The model under review builds one solid part; all positions refer to its coordinate system, in mm. A direction names the side the tool comes from. Coordinates: 2 decimals unless noted, no trailing zeros. Order: outer loops, then holes, each group sorted by start corner. A loop starts at its lowest first (then second) coordinate and runs counter-clockwise, first axis right, second up. Notation, with made-up numbers: M 4.5,89.5 L 13.5,89.5 A27 ccw 13.5,120.5 Z; hole C 82.5,44 d9. An arc over 180 degrees is marked long. Answer in a Markdown table with one row per item.
Autodesk Inventor part; units mm, degrees
ref_plane "YZ Plane" through (0, 0, 0) normal (1, 0, 0) x (0, 1, 0)
ref_plane "XZ Plane" through (0, 0, 0) normal (0, 1, 0) x (-1, 0, 0)
ref_plane "XY Plane" through (0, 0, 0) normal (0, 0, 1) x (1, 0, 0)
sketch "Sketch1" plane through (0, 0, 0) normal (0, 1, 0) x (-1, 0, 0)
  circle A0 centre (0, 0) radius 18.4566
  circle A1 centre (10, 10) radius 2
  circle A2 centre (10, -10) radius 2
  circle A3 centre (-10, -10) radius 2
  circle A4 centre (-10, 10) radius 2
  point P0 (8.8496, 0)
extrude "Extrusion1" add sketch "Sketch1" along normal blind 10
sketch "Sketch2" plane through (0, 10, 0) normal (0, 1, 0) x (1, 0, 0)
  circle A0 centre (0, 0) radius 10
  dimension "d2" = 20
extrude "Extrusion2" add sketch "Sketch2" along normal blind 14
sketch "Sketch3" plane through (0, 24, 0) normal (0, 1, 0) x (1, 0, 0)
  circle A0 centre (0, 0) radius 4
  dimension "d5" = 8
extrude "Extrusion3" cut sketch "Sketch3" against normal blind 14
sketch "Sketch4" plane through (0, 0, 0) normal (1, 0, 0) x (0, 1, 0)
  line L0 (24, -10) -> (24, 10)
  line L1 (24, 0) -> (17, 0)
  circle A0 centre (17, 0) radius 2
  point P0 (0, 0)
  dimension "d8" = 7
  dimension "d9" = 4
extrude "Extrusion4" cut sketch "Sketch4" against normal blind 14
sketch "Sketch5" plane through (0, 10, 0) normal (0, 1, 0) x (1, 0, 0)
  circle A0 centre (0, 0) radius 10
  circle A1 centre (0, 0) radius 18.4566
  circle A2 centre (10, -10) radius 2
  circle A3 centre (10, 10) radius 2
  circle A4 centre (-10, 10) radius 2
  circle A5 centre (-10, -10) radius 2
  circle A6 centre (-10, -10) radius 2
  circle A7 centre (-10, -10) radius 4.1421
  circle A8 centre (0, 0) radius 10
  circle A9 centre (-10, 10) radius 2
  circle A10 centre (-10, 10) radius 4.1421
properties part number "perilla"
(1) To check wall thickness, follow line 1 (X direction, y = 3.75, z = 9.5); line 2 (Z direction, x = -10, y = 6.25); line 3 (Y direction, x = 8.5, z = 6.5). State the ranges of each line that lie inside material, in increasing order. Write a range as [from, to].
Report:
| item | result |
|---|---|
| line 1 | [-15.82, -11.94], [-8.06, 8.06], [11.94, 15.82] |
| line 2 | [-15.51, -12], [-8, 8], [12, 15.51] |
| line 3 | [0, 10] |
(2) The part is to be moulded in two halves that separate along X. For faces 1 (the cylindrical face through (9.54, 16.9, 3)), 2 (the cylindrical face through (3.695, 17.098, 1.532)), 3 (the flat face through (-8, 10, -8)), say which applies: +X half, -X half, draft (parallel to the pull), parting line (faces both ways), or undercut.
Report:
| item | result |
|---|---|
| face 1 | parting line |
| face 2 | undercut |
| face 3 | draft |
(3) Insertion check: P1, Ø4, axis at x = -4.5, y = 11, coming from the +Z side; P2, Ø6, axis at x = -7.5, y = 3, coming from the +Z side; P3, Ø6.5, axis at x = 1, z = -0.5, coming from the +Y side; P4, Ø4.5, axis at x = -10, z = 10, coming from the +Y side. Each pin has a flat end and moves straight along its axis. Give the tip position at first contact, or say it passes through.
Report:
| item | result |
|---|---|
| P1 | z = 18.25 |
| P2 | z = 17.9 |
| P3 | y = 24 |
| P4 | y = 10 |
(4) Take a section at C-C (y = 17.25). Write out the cut boundary in (x, z), then the cut area to 3 significant figures.
Report:
| item | result |
|---|---|
| outline | M -9.8,-1.98 A10 ccw long -9.8,1.98 L -3.47,1.98 A4 cw long -3.47,-1.98 Z |
| area | 240 mm^2 |
(5) Take a section at D-D (x = -2.5). Write out the cut boundary in (y, z).
Report:
| item | result |
|---|---|
| outline | M 0,-18.29 L 10,-18.29 L 10,-9.68 L 24,-9.68 L 24,-3.12 L 10,-3.12 L 10,3.12 L 24,3.12 L 24,9.68 L 10,9.68 L 10,18.29 L 0,18.29 Z |
(6) Take a section at A-A (x = 5). Write out the cut boundary in (y, z), then the cut area to 3 significant figures.
Report:
| item | result |
|---|---|
| outline | M 0,-17.77 L 10,-17.77 L 10,-8.66 L 24,-8.66 L 24,8.66 L 10,8.66 L 10,17.77 L 0,17.77 Z |
| area | 598 mm^2 |
(7) Take a section at B-B (z = 2.5). Write out the cut boundary in (x, y), then the cut area to 3 significant figures.
Report:
| item | result |
|---|---|
| outline | M -18.29,0 L 18.29,0 L 18.29,10 L 9.68,10 L 9.68,24 L 3.12,24 L 3.12,10 L -3.12,10 L -3.12,24 L -9.68,24 L -9.68,10 L -18.29,10 Z |
| area | 549 mm^2 |
(8) Machinability: for faces 4 (the cylindrical face through (-7, 17, 2)), 5 (the flat face through (0, 10, 0)), 6 (the cylindrical face through (10, 5, -12)), which of the approach directions +Z, -Z, +X, -X, +Y, -Y give a long, thin tool a straight path to every point of the face, cutting with its end or side? Answer none if there is none.
Report:
| item | result |
|---|---|
| face 4 | -X |
| face 5 | +Y |
| face 6 | +Y, -Y |
